from build123d import *

# Parameters (mm, degrees)
SKETCH2_W           = 35
SKETCH2_H           = 27.6
BOSS_EXTRUDE1_DEPTH = 2.5
SKETCH3_W           = 12
SKETCH3_H           = 2.5
SKETCH3_W_2         = 4.8
SKETCH3_H_2         = 4
BOSS_EXTRUDE2_DEPTH = 11.8
SKETCH5_R           = 0.95
CUT_EXTRUDE2_DEPTH  = 11.8
SKETCH6_R           = 0.95
CUT_EXTRUDE3_DEPTH  = 11.8
CUT_EXTRUDE6_DEPTH  = 10
CHAMFER1_SIZE       = 1


with BuildPart() as part:
    # Sketch2 → Boss-Extrude1 (new body)
    with BuildSketch(Plane(origin=(0, 0, 0), x_dir=(1, 0, 0), z_dir=(0, 1, 0))):
        Rectangle(SKETCH2_W, SKETCH2_H)
    extrude(amount=BOSS_EXTRUDE1_DEPTH)

    # Sketch3 → Boss-Extrude2 (add)
    with BuildSketch(Plane.XZ):
        with Locations((6.7, -12.55)):
            Rectangle(SKETCH3_W, SKETCH3_H)
        with Locations((15.1, 11.8)):
            Rectangle(SKETCH3_W_2, SKETCH3_H_2)
        Polygon((-17.5, 13.8), (-15.2, 13.8), (-10.4, 13.8), (-10.4, 9.8), (-15.2, 9.8), (-15.2, -13.8), (-17.5, -13.8), align=None)
    extrude(amount=BOSS_EXTRUDE2_DEPTH)

    # Sketch5 → Cut-Extrude2 (cut)
    with BuildSketch(Plane(origin=(0, 0, -13.8), x_dir=(-1, 0, 0), z_dir=(0, 0, -1))):
        with Locations((-6.7, -6)):
            Circle(SKETCH5_R)
    extrude(amount=-CUT_EXTRUDE2_DEPTH, mode=Mode.SUBTRACT)

    # Sketch6 → Cut-Extrude3 (cut)
    with BuildSketch(Plane(origin=(0, 0, 9.8), x_dir=(-1, 0, 0), z_dir=(0, 0, -1))):
        with Locations((-15.1, -5.9)):
            Circle(SKETCH6_R)
        with Locations((12.8, -5.9)):
            Circle(SKETCH6_R)
    extrude(amount=-CUT_EXTRUDE3_DEPTH, mode=Mode.SUBTRACT)

    # Sketch11 → Cut-Extrude6 (cut)
    with BuildSketch(Plane(origin=(0, 0, 0), x_dir=(-1, 0, 0), z_dir=(0, -1, 0))):
        Polygon((-12.7, 13.8), (-17.5, -9.8), (-17.5, 13.8), align=None)
        Polygon((-12.909628956, -7.3), (-9.7367476, 8.3), (12.2, 8.3), (12.2, -7.3), align=None)
    extrude(amount=-CUT_EXTRUDE6_DEPTH, mode=Mode.SUBTRACT)

    # Chamfer1
    chamfer1_edges = [part.edges().sort_by_distance(p)[0] for p in [
        (17.5, 2.5, 11.8),
    ]]
    chamfer(chamfer1_edges, length=CHAMFER1_SIZE)


solid = part.part
Can you work these out from the model? Positions are in its coordinate system, mm. A direction names the side the tool comes from. Give positions to 0.01 mm unless a question says otherwise; leave off trailing zeros. Order: outer loops, then holes, each group sorted by start corner. A loop starts at its lowest first (then second) coordinate and runs counter-clockwise, first axis right, second up. Notation, with made-up numbers: (48, 35.5) - (97, 35.5) arc R30 cw to (97, 57.5) - close; hole circle Ø5 at (53.5, 82.25). An arc over 180 degrees is marked (long way). Write each question's results on one line, items separated by ' | '.
1) On a 3-axis mill with a long thin cutter (end or side, diameter ignored), from which of +Z, -Z, +X, -X, +Y, -Y can I reach the whole of each face in a straight line? I mean faces 4 (the face through (0, 1, 7.3)), 5 (the face through (12.7, -6, 12)), 6 (the face through (-10.4, -6, 12)), 7 (the face through (12.7, -6, -13)). Say none if no direction works.
Final values:
face 4: +Y, -Y | face 5: +Z, -Y | face 6: +Z, -Z, -Y | face 7: -Z, +X, -Y
2) I'm going to push flat-ended pins straight in: pin 1 Ø2.5 at (x, y) = (16, -5.5) entering from -Z; pin 2 Ø1.2 at (y, z) = (-5, -13) entering from +X; pin 3 Ø5 at (y, z) = (-5, -8.5) entering from +X; pin 4 Ø3 at (x, y) = (6.7, -6) entering from -Z. Where does each tip first touch, or does it pass through?
Final values:
pin 1: stops at z = 9.8 | pin 2: stops at x = 12.7 | pin 3: stops at x = -15.2 | pin 4: stops at z = -13.8
3) Please list where these lines run through material, in increasing order: line 1 along Y through (x, z) = (6.7, -12.5); line 2 along X through (y, z) = (-8.25, -12.25); line 3 along Z through (x, y) = (-9, 1). Write a range as [from, to].
Final values:
line 1: y = [-11.8, -6.95], [-5.05, 2.5] | line 2: x = [-17.5, -15.2], [0.7, 12.7] | line 3: z = [-13.8, -8.3], [7.3, 13.8]
4) Suppose I cut it at A-A, the plane x = 0. Write out the boundary of the cut face in (y, z), then the cut area to 3 significant figures.
Final values:
outline: (0, -13.8) - (2.5, -13.8) - (2.5, -8.3) - (0, -8.3) - close; (0, 7.3) - (2.5, 7.3) - (2.5, 13.8) - (0, 13.8) - close | area: 30.0 mm^2
5) If we mould it in two halves opening along Y, with no side actions, what happens to faces 1 (the face through (7, -11.8, -13)), 2 (the face through (6.26, -6.84, -12.57)), 3 (the face through (-15.2, -6, -2))? For each: pulls with the +Y half, pulls with the -Y half, needs draft (parallel to the pull), parting line crosses it, or undercut.
Final values:
face 1: pulls with the -Y half | face 2: undercut | face 3: needs draft
6) Suppose I cut it at D-D, the plane x = -12.8. Write out the boundary of the cut face in (y, z), then the cut area to 3 significant figures.
Final values:
outline: (-11.8, 9.8) - (-6.85, 9.8) - (-6.85, 13.8) - (-11.8, 13.8) - close; (-4.95, 9.8) - (0, 9.8) - (0, -13.8) - (2.5, -13.8) - (2.5, 13.8) - (-4.95, 13.8) - close | area: 109 mm^2
7) Suppose I cut it at B-B, the plane y = -2.25. Write out the boundary of the cut face in (x, z), then the cut area to 3 significant figures.
Final values:
outline: (-17.5, -13.8) - (-15.2, -13.8) - (-15.2, 9.8) - (-10.4, 9.8) - (-10.4, 13.8) - (-17.5, 13.8) - close; (0.7, -13.8) - (12.7, -13.8) - (12.7, -11.3) - (0.7, -11.3) - close; (12.7, 9.8) - (17.5, 9.8) - (17.5, 13.8) - (12.7, 13.8) - close | area: 132 mm^2
8) Suppose I cut it at C-C, the plane z = 3. Write out the boundary of the cut face in (x, y), then the cut area to 3 significant figures.
Final values:
outline: (-17.5, -11.8) - (-15.2, -11.8) - (-15.2, 0) - (-12.2, 0) - (-12.2, 2.5) - (-17.5, 2.5) - close; (12.04, 0) - (16.12, 0) - (16.12, 2.5) - (12.04, 2.5) - close | area: 50.6 mm^2
